Autodesk Inventor part; units mm, degrees
ref_plane "YZ Plane" through (0, 0, 0) normal (1, 0, 0) x (0, 1, 0)
ref_plane "XZ Plane" through (0, 0, 0) normal (0, 1, 0) x (-1, 0, 0)
ref_plane "XY Plane" through (0, 0, 0) normal (0, 0, 1) x (1, 0, 0)
sketch "Эскиз1" plane through (0, 0, 0) normal (0, 0, 1) x (1, 0, 0)
  line L0 (28.5, 35) -> (-28.5, 35)
  arc A0 (32.5, 31) -> (28.5, 35) centre (28.5, 31) ccw
  arc A1 (-28.5, 35) -> (-32.5, 31) centre (-28.5, 31) ccw
  line L1 (-32.5, 31) -> (-32.5, -35)
  line L2 (32.5, -35) -> (32.5, 31)
  line L3 (26.5, -35) -> (32.5, -35)
  line L4 (-32.5, -35) -> (-26.5, -35)
  line L5 (26.5, -35) -> (-26.5, -35)
  point P0 (0, 0)
extrude "Выдавливание1" add sketch "Эскиз1" along normal blind 3
ref_plane "РабПлоскость1" through (26.5, -31, -4) normal (-1, 0, 0) x (0, -1, 0)
sketch "Эскиз3" plane through (26.5, -31, -4) normal (-1, 0, 0) x (0, -1, 0)
  line L0 (-4, 4) -> (-4, -4)
  line L1 (-4, -4) -> (4, -4)
  line L2 (4, -4) -> (4, 4)
  line L3 (4, 4) -> (-4, 4)
  circle A0 centre (0, 0) radius 1.95
  point P0 (-31, 4)
extrude "Выдавливание3" add sketch "Эскиз3" along normal blind 5
sketch "Эскиз4" plane through (-32.5, -35, 3) normal (0, -1, 0) x (1, 0, 0)
  line L0 (0, -79.5) -> (0, -3)
  line L1 (0, -3) -> (0, 0)
  line L2 (0, 0) -> (65, 0)
  line L3 (65, -3) -> (65, 0)
  line L4 (65, -79.5) -> (65, -3)
  arc A0 (61, -83.5) -> (65, -79.5) centre (61, -79.5) ccw
  line L5 (4, -83.5) -> (61, -83.5)
  arc A1 (0, -79.5) -> (4, -83.5) centre (4, -79.5) ccw
  point P0 (32.5, -3)
extrude "Выдавливание4" add sketch "Эскиз4" along normal blind 3
ref_plane "РабПлоскость3" through (0, 31, 0) normal (-1, 0, 0) x (0, 0, 1)
mirror "Зеркальное отражение2" about plane through (0, 31, 0) normal (-1, 0, 0) of "Выдавливание3"
fillet "Сопряжение3" radius 4 1 edges at (0, -38, 3)
properties part number "tail_box_cup"
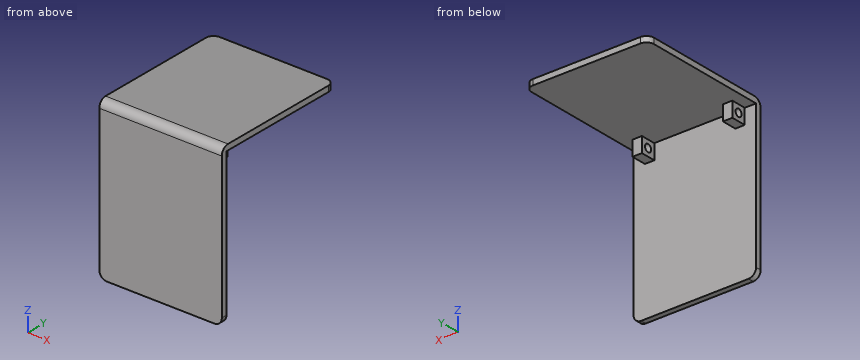
Source: CAD feature listing. Evaluate the final solid. Frame: model axes, mm. Coordinates: 2 decimals unless noted, no trailing zeros. Loops run counter-clockwise (first coordinate to the right, second up) from the corner with the lowest first, then second, coordinate; pieces in that order, holes last. Notation, with made-up numbers: (-5.75, 38.5) -> (4.25, 38.5) arc R18 ccw to (4.25, 63.5) -> close; hole circle Ø1 at (57, 29). An arc over 180 degrees is marked (long way). One line per item, written item: value. Start each with the question number.
Q1. Line query: line 1 along Z through (x, y) = (-23, -31); line 2 along Z through (x, y) = (-2.5, 9); line 3 along Y through (x, z) = (-4, -65). Output: solid intervals per line, ascending.
Q2. Section query C-C, the plane x = 25. Return the cut outline in (y, z), and give its area (3 significant figures).
Q3. Contact query for flat-ended pins moving along their axis: P1, Ø1.5, axis at x = 24.5, z = -3, coming from the +Y side; P2, Ø6, axis at y = -31, z = -4, coming from the -X side; P3, Ø12, axis at x = 13.5, y = -27.5, coming from the -Z side. Output: stop coordinate, or through.
Q4. Section query A-A, the plane z = -4. Return the cut outline in (x, y).
Q5. Section query D-D, the plane x = -9. Return the cut outline in (y, z).
Q6. Section query B-B, the plane y = -31. Return the cut outline in (x, z), and give its area (3 significant figures).
Results:
1. line 1: -8 to -5.95, -2.05 to 3
1. line 2: 0 to 3
1. line 3: -38 to -35
2. outline: (-38, -80.5) -> (-35, -80.5) -> (-35, -8) -> (-27, -8) -> (-27, 0) -> (35, 0) -> (35, 3) -> (-34, 3) arc R4 ccw to (-38, -1) -> close; hole circle Ø3.9 at (-31, -4)
2. area: 509 mm^2
3. P1: y = -27
3. P2: x = -26.5
3. P3: z = 0
4. outline: (-32.5, -38) -> (32.5, -38) -> (32.5, -35) -> (26.5, -35) -> (26.5, -32.95) -> (21.5, -32.95) -> (21.5, -35) -> (-21.5, -35) -> (-21.5, -32.95) -> (-26.5, -32.95) -> (-26.5, -35) -> (-32.5, -35) -> close; (-26.5, -29.05) -> (-21.5, -29.05) -> (-21.5, -27) -> (-26.5, -27) -> close; (21.5, -29.05) -> (26.5, -29.05) -> (26.5, -27) -> (21.5, -27) -> close
5. outline: (-38, -80.5) -> (-35, -80.5) -> (-35, 0) -> (35, 0) -> (35, 3) -> (-34, 3) arc R4 ccw to (-38, -1) -> close
6. outline: (-32.5, 0) -> (-26.5, 0) -> (-26.5, -2.05) -> (-21.5, -2.05) -> (-21.5, 0) -> (21.5, 0) -> (21.5, -2.05) -> (26.5, -2.05) -> (26.5, 0) -> (32.5, 0) -> (32.5, 3) -> (-32.5, 3) -> close; (-26.5, -8) -> (-21.5, -8) -> (-21.5, -5.95) -> (-26.5, -5.95) -> close; (21.5, -8) -> (26.5, -8) -> (26.5, -5.95) -> (21.5, -5.95) -> close
6. area: 236 mm^2
